from build123d import *

# Parameters (mm, degrees)
SKETCH1_R                            = 5.08
BOSS_EXTRUDE1_DEPTH                  = 88.9
TAPPED_HOLE_FOR_4_40_HELICOIL1_D     = 3.048
TAPPED_HOLE_FOR_4_40_HELICOIL1_DEPTH = 8.128
TAPPED_HOLE_FOR_4_40_HELICOIL1_TIP   = 0.915711583
TAPPED_HOLE_FOR_4_40_HELICOIL2_D     = 3.048
TAPPED_HOLE_FOR_4_40_HELICOIL2_DEPTH = 8.128
TAPPED_HOLE_FOR_4_40_HELICOIL2_TIP   = 0.915711583


with BuildPart() as part:
    # Sketch1 → Boss-Extrude1 (new body)
    with BuildSketch(Plane(origin=(0, 0, 0), x_dir=(1, 0, 0), z_dir=(0, 1, 0))):
        with Locations(Location((0, 0, 0), (0, 0, 270))):
            Circle(SKETCH1_R)
    extrude(amount=BOSS_EXTRUDE1_DEPTH)

    # Tapped Hole for #4-40 Helicoil1
    with Locations(Plane(origin=(0, 88.9, 0), x_dir=(1, 0, 0), z_dir=(0, 1, 0))):
        with Locations((0, 0)):
            Hole(TAPPED_HOLE_FOR_4_40_HELICOIL1_D / 2, depth=TAPPED_HOLE_FOR_4_40_HELICOIL1_DEPTH)
            with Locations((0, 0, -(TAPPED_HOLE_FOR_4_40_HELICOIL1_DEPTH + TAPPED_HOLE_FOR_4_40_HELICOIL1_TIP / 2))):  # 118° drill point
                Cone(0, TAPPED_HOLE_FOR_4_40_HELICOIL1_D / 2, TAPPED_HOLE_FOR_4_40_HELICOIL1_TIP, mode=Mode.SUBTRACT)

    # Tapped Hole for #4-40 Helicoil2
    with Locations(Plane(origin=(0, 0, 0), x_dir=(-1, 0, 0), z_dir=(0, -1, 0))):
        with Locations((0, 0)):
            Hole(TAPPED_HOLE_FOR_4_40_HELICOIL2_D / 2, depth=TAPPED_HOLE_FOR_4_40_HELICOIL2_DEPTH)
            with Locations((0, 0, -(TAPPED_HOLE_FOR_4_40_HELICOIL2_DEPTH + TAPPED_HOLE_FOR_4_40_HELICOIL2_TIP / 2))):  # 118° drill point
                Cone(0, TAPPED_HOLE_FOR_4_40_HELICOIL2_D / 2, TAPPED_HOLE_FOR_4_40_HELICOIL2_TIP, mode=Mode.SUBTRACT)


solid = part.part
Work out the finished part from the listing and answer in its coordinate system (mm). A direction names the side the tool comes from. Give positions to 0.01 mm unless a question says otherwise; leave off trailing zeros. Write each loop counter-clockwise with the first axis right and the second up, starting at its lowest first coordinate (ties: lowest second). Pieces come first, ordered by that corner, then holes.
Q1. A tool of negligible diameter and unlimited length cuts with its end or side. For faces 4 (the face through (1.2, 0, -1.2)), 5 (the face through (0.2, 84.78, -1.51)), from which of +Z, -Z, +X, -X, +Y, -Y can it reach the whole face along a straight path? Write none if from no direction.
Answer:
face 4: +Z, -Z, +X, -X, -Y
face 5: +Y
Q2. The part is cut by section A-A on y = 42. Give the vertices of the cut face in (x, z).
Answer:
outline: circle Ø10.16 at (0, 0)
Q3. Given pin 1 (1.5 mm diameter, centred on y = 24.5, z = -4, fed in from -X); pin 2 (3 mm diameter, centred on y = 75.5, z = 3.5, fed in from -X); pin 3 (1.8 mm diameter, centred on x = 0, z = 0, fed in from +Y); pin 4 (6 mm diameter, centred on x = 3, z = -1, fed in from -Y), each flat-ended and moving along its own axis, determine where each tip first touches the part or whether it passes through.
Answer:
pin 1: stops at x = -3.9
pin 2: stops at x = -4.67
pin 3: stops at y = 80.4
pin 4: stops at y = 0
Q4. Straight lines are drawn through the part: L1, parallel to Z at x = -0.25, y = 24; L2, parallel to X at y = 10, z = 1.25; L3, parallel to Z at x = 1.75, y = 21. For each, find the intervals that lie inside material, in ascending order.
Answer:
L1: z = -5.07 to 5.07
L2: x = -4.92 to 4.92
L3: z = -4.77 to 4.77
Q5. The part is cut by section B-B on z = 3.25. Give the vertices of the cut face in (x, y), and give its area (3 significant figures).
Answer:
outline: (-3.9, 0) - (3.9, 0) - (3.9, 88.9) - (-3.9, 88.9) - close
area: 694 mm2
Q6. The part is cut by section C-C on x = -3. Give the vertices of the cut face in (y, z), and give its area (3 significant figures).
Answer:
outline: (0, -4.1) - (88.9, -4.1) - (88.9, 4.1) - (0, 4.1) - close
area: 729 mm2
Q7. For a pull along Z with two mould halves and no side action, classify faces 1 (the face through (-0.2, 4.12, -1.51)), 2 (the face through (1.2, 88.9, -1.2)), 3 (the face through (5.037, 43.828, -0.661)) as released by +Z, released by -Z, zero draft, split by the parting line, or undercut.
Answer:
face 1: undercut
face 2: zero draft
face 3: split by the parting line
